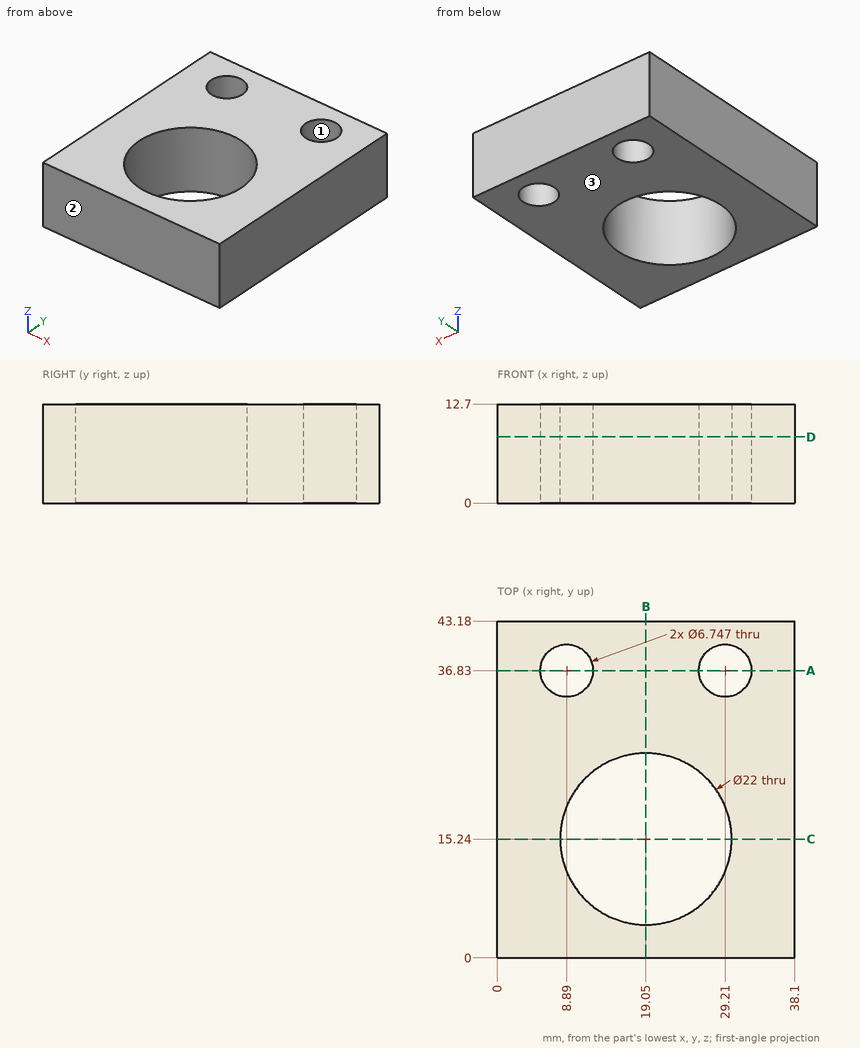
Part print with two shaded views. Sizes in mm from the minimum x, y, z corner. Round coordinates to 2 decimals unless told otherwise and drop trailing zeros. Write each loop counter-clockwise with the first axis right and the second up, starting at its lowest first coordinate (ties: lowest second). Pieces come first, ordered by that corner, then holes. Notation, with made-up numbers: M 86.25,51 L 139.25,51 A23 cw 139.25,72 Z; hole C 0,46 d3. An arc over 180 degrees is marked long. Put each result on its own line as item: value. Start each with the question number.
1) Saw through at A-A, the plane y = 36.83. Write the cut outline in (x, z).
2) Saw through at B-B, the plane x = 19.05. Write the cut outline in (y, z), and give its area (3 significant figures).
3) Pull direction Y, two halves, no side cores. Call the marked faces 1, 2 and 3: pulls with the +Y half, pulls with the -Y half, needs draft (parallel to the pull), parting line crosses it, or undercut.
4) Drill centre lines: probe 1 along Y at (x, z) = (29.21, 7.25); probe 2 along X at (y, z) = (36, 6); probe 3 along Y at (x, z) = (10, 11). Where is each one in solid material? Low to high. Write a range as [from, to].
5) Saw through at C-C, the plane y = 15.24. Write the cut outline in (x, z).
6) Pin check, flat tips, straight feed: pin 1 Ø5.5 at (x, y) = (29.21, 36.83) entering from +Z; pin 2 Ø4 at (y, z) = (25, 9.5) entering from -X. Stop position of each tip, or through.
7) Saw through at D-D, the plane z = 8.5. Write the cut outline in (x, y), and give its area (3 significant figures).
Resolved:
1. outline: M 0,0 L 5.52,0 L 5.52,12.7 L 0,12.7 Z; M 12.26,0 L 25.84,0 L 25.84,12.7 L 12.26,12.7 Z; M 32.58,0 L 38.1,0 L 38.1,12.7 L 32.58,12.7 Z
2. outline: M 0,0 L 4.24,0 L 4.24,12.7 L 0,12.7 Z; M 26.24,0 L 43.18,0 L 43.18,12.7 L 26.24,12.7 Z
2. area: 269 mm²
3. face 1: undercut
3. face 2: pulls with the -Y half
3. face 3: needs draft
4. probe 1: [0, 11.02], [19.46, 33.46], [40.2, 43.18]
4. probe 2: [0, 5.62], [12.16, 25.94], [32.48, 38.1]
4. probe 3: [0, 8.99], [21.49, 33.64], [40.02, 43.18]
5. outline: M 0,0 L 8.05,0 L 8.05,12.7 L 0,12.7 Z; M 30.05,0 L 38.1,0 L 38.1,12.7 L 30.05,12.7 Z
6. pin 1: through
6. pin 2: x = 0
7. outline: M 0,0 L 38.1,0 L 38.1,43.18 L 0,43.18 Z; hole C 8.89,36.83 d6.75; hole C 19.05,15.24 d22; hole C 29.21,36.83 d6.75
7. area: 1,190 mm²
